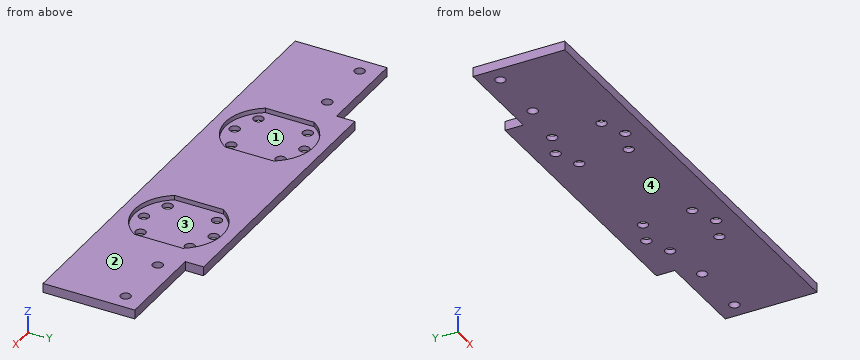
from build123d import *

# Parameters (mm, degrees)
SKETCH_1_W          = 290
SKETCH_1_H          = 50
EXTRUDE_1_DEPTH     = 5
SKETCH_3_W          = 20
SKETCH_3_H          = 50
CUT_EXTRUDE_1_DEPTH = 10
SKETCH_4_W          = 150
SKETCH_4_H          = 5
EXTRUDE_2_DEPTH     = 10
SKETCH_2_R          = 2.75
CUT_EXTRUDE_2_DEPTH = 2.5
SKETCH_2_2_R        = 2.75
CUT_EXTRUDE_3_DEPTH = 130.903810568
SKETCH_5_R          = 2.75
CUT_EXTRUDE_4_DEPTH = 130.903810568


with BuildPart() as part:
    # Sketch 1 → Extrude 1 (new body)
    with BuildSketch(Plane.XY):
        Rectangle(SKETCH_1_W, SKETCH_1_H)
    extrude(amount=EXTRUDE_1_DEPTH)

    # Sketch 3 → Cut-Extrude 1 (cut)
    with BuildSketch(Plane.XY.offset(5)):
        with Locations((-135, 0)):
            Rectangle(SKETCH_3_W, SKETCH_3_H)
    cut_extrude_1 = extrude(amount=-CUT_EXTRUDE_1_DEPTH, mode=Mode.SUBTRACT)

    # Mirror 1: Cut-Extrude 1 across plane
    add(cut_extrude_1.mirror(Plane(origin=(0, 0, 0), x_dir=(0, 0, 1), z_dir=(1, 0, 0))), mode=Mode.SUBTRACT)

    # Sketch 4 → Extrude 2 (add)
    with BuildSketch(Plane(origin=(0, 25, 0), x_dir=(1, 0, 0), z_dir=(0, 1, 0))):
        with Locations((0, -2.5)):
            Rectangle(SKETCH_4_W, SKETCH_4_H)
    extrude(amount=EXTRUDE_2_DEPTH)

    # Sketch 2 → Cut-Extrude 2 (cut)
    # profile 1 of 2: a face of its own
    with BuildSketch(Plane.XY.offset(5)):
        with BuildLine():
            Line((65, 18.26), (65, -8.27))
            ThreePointArc((65, -8.27), (45.000804497, -19.004999933), (25, -8.272998079))
            Line((25, -8.272998079), (25, 18.262998079))
            ThreePointArc((25, 18.262998079), (45.000804497, 28.994999933), (65, 18.26))
        make_face()
        with Locations((58.44, -8.437)):
            Circle(SKETCH_2_R, mode=Mode.SUBTRACT)
        with Locations(Location((31.558011299, -8.437, 0), (0, 0, 180))):
            Circle(SKETCH_2_R, mode=Mode.SUBTRACT)
        with Locations((44.99900565, -14)):
            Circle(SKETCH_2_R, mode=Mode.SUBTRACT)
        with Locations(Location((58.44, 18.427, 0), (0, 0, 180))):
            Circle(SKETCH_2_R, mode=Mode.SUBTRACT)
        with Locations(Location((44.99900565, 23.99, 0), (0, 0, 180))):
            Circle(SKETCH_2_R, mode=Mode.SUBTRACT)
        with Locations((31.558011299, 18.427)):
            Circle(SKETCH_2_R, mode=Mode.SUBTRACT)
    # profile 2 of 2: a face of its own
    with BuildSketch(Plane.XY.offset(5)):
        with BuildLine():
            Line((-25, 18.262998079), (-25, -8.272998079))
            ThreePointArc((-25, -8.272998079), (-45.000804497, -19.004999933), (-65, -8.27))
            Line((-65, -8.27), (-65, 18.26))
            ThreePointArc((-65, 18.26), (-45.000804497, 28.994999933), (-25, 18.262998079))
        make_face()
        with Locations(Location((-31.558011299, 18.427, 0), (0, 0, 180))):
            Circle(SKETCH_2_R, mode=Mode.SUBTRACT)
        with Locations((-44.99900565, 23.99)):
            Circle(SKETCH_2_R, mode=Mode.SUBTRACT)
        with Locations((-58.44, 18.427)):
            Circle(SKETCH_2_R, mode=Mode.SUBTRACT)
        with Locations(Location((-44.99900565, -14, 0), (0, 0, 180))):
            Circle(SKETCH_2_R, mode=Mode.SUBTRACT)
        with Locations((-31.558011299, -8.437)):
            Circle(SKETCH_2_R, mode=Mode.SUBTRACT)
        with Locations(Location((-58.44, -8.437, 0), (0, 0, 180))):
            Circle(SKETCH_2_R, mode=Mode.SUBTRACT)
    extrude(amount=-CUT_EXTRUDE_2_DEPTH, mode=Mode.SUBTRACT)

    # Sketch 2_2 → Cut-Extrude 3 (cut, through all)
    with BuildSketch(Plane.XY.offset(5)):
        with Locations((-58.44, 18.427)):
            Circle(SKETCH_2_2_R)
        with Locations((-44.99900565, 23.99)):
            Circle(SKETCH_2_2_R)
        with Locations((-31.558011299, 18.427)):
            Circle(SKETCH_2_2_R)
        with Locations((-58.44, -8.437)):
            Circle(SKETCH_2_2_R)
        with Locations((-44.99900565, -14)):
            Circle(SKETCH_2_2_R)
        with Locations((-31.558011299, -8.437)):
            Circle(SKETCH_2_2_R)
        with Locations((58.44, -8.437)):
            Circle(SKETCH_2_2_R)
        with Locations((58.44, 18.427)):
            Circle(SKETCH_2_2_R)
        with Locations((44.99900565, 23.99)):
            Circle(SKETCH_2_2_R)
        with Locations((31.558011299, 18.427)):
            Circle(SKETCH_2_2_R)
        with Locations(Location((31.558011299, -8.437, 0), (0, 0, 180))):
            Circle(SKETCH_2_2_R)
        with Locations((44.99900565, -14)):
            Circle(SKETCH_2_2_R)
    extrude(amount=-CUT_EXTRUDE_3_DEPTH, mode=Mode.SUBTRACT)

    # Sketch 5 → Cut-Extrude 4 (cut, through all)
    with BuildSketch(Plane.XY.offset(5)):
        with Locations((-84, 15)):
            Circle(SKETCH_5_R)
        with Locations((-116, 15)):
            Circle(SKETCH_5_R)
        with Locations(Location((116, 15, 0), (0, 0, 180))):
            Circle(SKETCH_5_R)
        with Locations(Location((84, 15, 0), (0, 0, 180))):
            Circle(SKETCH_5_R)
    extrude(amount=-CUT_EXTRUDE_4_DEPTH, mode=Mode.SUBTRACT)


solid = part.part
Verification items for the finished model (mm, model axes). Face numbers are marked on the shaded views. A direction names the side the tool comes from. Coordinates: 2 decimals unless noted, no trailing zeros. Order: outer loops, then holes, each group sorted by start corner. A loop starts at its lowest first (then second) coordinate and runs counter-clockwise, first axis right, second up. Notation, with made-up numbers: M -29,-22.75 L 4,-22.75 A13 cw 4,-13.75 Z; hole C 24,82.25 d11. An arc over 180 degrees is marked long. Return JSON: item names as keys, results as strings.
1) Cross-section at D-D, the plane x = -51. Record the boundary of the cut face in (y, z).
Answer list:
{"outline": "M -25,0 L 35,0 L 35,5 L 28.23,5 L 28.23,2.5 L -18.24,2.5 L -18.24,5 L -25,5 Z"}
2) Cross-section at A-A, the plane x = 116. Record the boundary of the cut face in (y, z), and give its area (4 significant figures).
Answer list:
{"outline": "M -25,0 L 12.25,0 L 12.25,5 L -25,5 Z; M 17.75,0 L 25,0 L 25,5 L 17.75,5 Z", "area": "222.5 mm2"}
3) Cross-section at B-B, the plane z = 4.25. Record the boundary of the cut face in (x, y) (3 decimals).
Answer list:
{"outline": "M -125,-25 L 125,-25 L 125,25 L 75,25 L 75,35 L -75,35 L -75,25 L -125,25 Z; hole C -116,15 d5.5; hole C -84,15 d5.5; hole M -65,-8.27 A24 ccw -25,-8.273 L -25,18.263 A24 ccw -65,18.26 Z; hole M 25,-8.273 A24 ccw 65,-8.27 L 65,18.26 A24 ccw 25,18.263 Z; hole C 84,15 d5.5; hole C 116,15 d5.5"}
4) Cross-section at C-C, the plane x = 58.44. Record the boundary of the cut face in (y, z), and give its area (3 significant figures).
Answer list:
{"outline": "M -25,0 L -11.19,0 L -11.19,2.5 L -14.89,2.5 L -14.89,5 L -25,5 Z; M -5.69,0 L 15.68,0 L 15.68,2.5 L -5.69,2.5 Z; M 21.18,0 L 35,0 L 35,5 L 24.88,5 L 24.88,2.5 L 21.18,2.5 Z", "area": "173 mm2"}
5) Release check for a two-part mould opening along X. For the marked faces 1 and 2 record: +X half, -X half, draft (parallel to the pull), parting line (faces both ways), or undercut.
Answer list:
{"face 1": "undercut", "face 2": "draft"}
6) Thickness scan on L1, parallel to X at y = -4, z = 4.4; L2, parallel to Y at x = 58.44, z = 0.75; L3, parallel to X at y = -14.5, z = 2.25. Record the ranges inside material, lowest first. Write a range as [from, to].
Answer list:
{"L1": "[-125, -65], [-25, 25], [65, 125]", "L2": "[-25, -11.19], [-5.69, 15.68], [21.18, 35]", "L3": "[-125, -47.7], [-42.29, 42.29], [47.7, 125]"}
7) Gauge pin test, flat ends, axial feed: pin 1 (3.5 mm diameter, centred on x = -58.44, y = 18.427, fed in from -Z); pin 2 (1.5 mm diameter, centred on y = 31.5, z = 3.5, fed in from -X); pin 3 (20 mm diameter, centred on x = 36, y = -1.5, fed in from +Z); pin 4 (1.5 mm diameter, centred on x = 95, z = 2, fed in from +Y). Record the tip position at first contact, or that the pin passes through.
Answer list:
{"pin 1": "through", "pin 2": "x = -75", "pin 3": "z = 2.5", "pin 4": "y = 25"}
8) Access from +Z, -Z, +X, -X, +Y, -Y to the whole of each face (thin tool, end or side, straight path). Record for the marked faces 3 and 4.
Answer list:
{"face 3": "+Z", "face 4": "-Z, +X, -X, +Y, -Y"}
